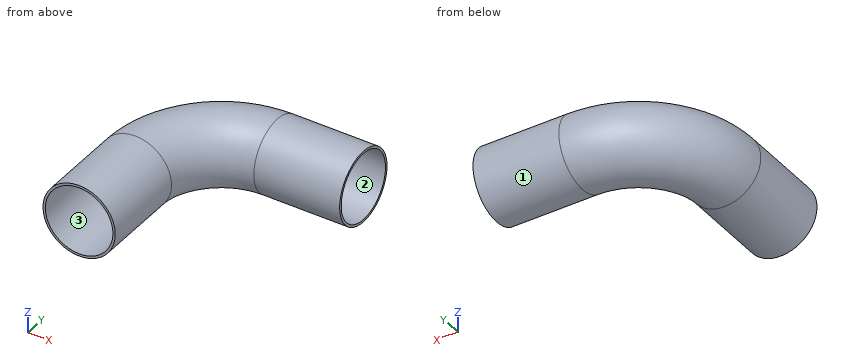
Autodesk Inventor part; units mm, degrees
ref_plane "YZ Plane" through (0, 0, 0) normal (1, 0, 0) x (0, 1, 0)
ref_plane "XZ Plane" through (0, 0, 0) normal (0, 1, 0) x (-1, 0, 0)
ref_plane "XY Plane" through (0, 0, 0) normal (0, 0, 1) x (1, 0, 0)
sketch "Sketch1" plane through (0, 0, 0) normal (0, 0, 1) x (1, 0, 0)
  line L0 (0, 0) -> (0, 60.35)
  line L1 (60.35, 120.7) -> (120.7, 120.7)
  arc A0 (60.35, 120.7) -> (0, 60.35) centre (60.35, 60.35) ccw
  dimension "d0" = 120.7
  dimension "d1" = 120.7
  dimension "d2" = 60.35
sketch "Sketch2" plane through (0, 0, 0) normal (0, 1, 0) x (-1, 0, 0)
  circle A0 centre (0, 0) radius 25.4
  circle A1 centre (0, 0) radius 23.75
  dimension "d4" = 1.65
  dimension "d5" = 50.8
sweep "Sweep1" add profiles "Sketch2" path "Sketch1"
equation "\"d1\" = d0"
equation "\"d2\" = 0.5 * d0"
properties part number "ASME BPE 90DEG ELB-50.8"
Geometry: final body of the model. Coordinates: model frame, mm. Face numbers are marked on the shaded views. Round coordinates to 2 decimals unless told otherwise and drop trailing zeros. Loops run counter-clockwise (first coordinate to the right, second up) from the corner with the lowest first, then second, coordinate; pieces in that order, holes last. Notation, with made-up numbers: (-10, -5) -> (19, -5) arc R23 ccw to (19, 31) -> close; hole circle Ø3 at (86, -7.75). An arc over 180 degrees is marked (long way). One line per question, with ' | ' between items. Start each with the question number.
1. Contact query for flat-ended pins moving along their axis: pin 1 (2 mm diameter, centred on x = 10.5, z = 1, fed in from -Y); pin 2 (1 mm diameter, centred on x = 27.5, z = 2.5, fed in from +Y); pin 3 (1.5 mm diameter, centred on x = 76.5, z = 11.5, fed in from +Y). Output: stop coordinate, or through.
2. Line query: line 1 along X through (y, z) = (37, 1); line 2 along Z through (x, y) = (102, 120); line 3 along Y through (x, z) = (82, 0). Output: solid intervals per line, ascending. Write a range as [from, to].
3. Section A-A on z = 0. Output: boundary loops of the cut face in (x, y), and give its area (3 significant figures).
4. Mould query, pull axis Y, two halves, no side actions, for the marked faces 1, 2 and 3. Classes: pulls with the +Y half, pulls with the -Y half, needs draft (parallel to the pull), parting line crosses it, or undercut.
5. Section B-B on z = -16.5. Output: boundary loops of the cut face in (x, y).
Returned:
1) pin 1: stops at y = 127.31 | pin 2: stops at y = 139.64 | pin 3: stops at y = 143.71
2) line 1: x = [-25.38, -23.73], [23.73, 25.38] | line 2: z = [-25.39, -23.74], [23.74, 25.39] | line 3: y = [95.3, 96.95], [144.45, 146.1]
3) outline: (-25.4, 0) -> (-23.75, 0) -> (-23.75, 60.35) arc R84.1 cw to (60.35, 144.45) -> (120.7, 144.45) -> (120.7, 146.1) -> (60.35, 146.1) arc R85.75 ccw to (-25.4, 60.35) -> close; (23.75, 0) -> (25.4, 0) -> (25.4, 60.35) arc R34.95 cw to (60.35, 95.3) -> (120.7, 95.3) -> (120.7, 96.95) -> (60.35, 96.95) arc R36.6 ccw to (23.75, 60.35) -> close | area: 711 mm2
4) face 1: parting line crosses it | face 2: undercut | face 3: needs draft
5) outline: (-19.31, 0) -> (-17.08, 0) -> (-17.08, 60.35) arc R77.43 cw to (60.35, 137.78) -> (120.7, 137.78) -> (120.7, 140.01) -> (60.35, 140.01) arc R79.66 ccw to (-19.31, 60.35) -> close; (17.08, 0) -> (19.31, 0) -> (19.31, 60.35) arc R41.04 cw to (60.35, 101.39) -> (120.7, 101.39) -> (120.7, 103.62) -> (60.35, 103.62) arc R43.27 ccw to (17.08, 60.35) -> close
